Check sheet for the modelled part. Datum: model origin and axes. Units: mm. Round coordinates to 2 decimals unless told otherwise and drop trailing zeros. Order: outer loops, then holes, each group sorted by start corner. A loop starts at its lowest first (then second) coordinate and runs counter-clockwise, first axis right, second up.
Q1. Mould release check, pull along X, two halves, no side actions. Record for faces 1 (the flat face through (1, -2.4, 1)), 2 (the conical face through (1.44, -0.09, -2.52)), 3 (the cylindrical face through (1.2, -1.18, -0.27)): +X half, -X half, draft (parallel to the pull), parting line (faces both ways), or undercut.
Q2. Scan lines: probe 1 along Z at (x, y) = (-1, -1.2); probe 2 along X at (y, z) = (-1, 0.45); probe 3 along Z at (x, y) = (-2.5, -0.9). Record each from-to range of solid material in increasing order.
Q3. Cross-section at A-A on y = -1.1. Record the cut outline in (x, z).
from build123d import *

# Parameters (mm, degrees)
SCHNITT_LINEAR_START            = -1e-07
SCHNITT_LINEAR_AUSTRAGEN1_DEPTH = 2.399991326


# Read off the part's stored shape, not the designer's step: Schnitt-Linear austragen1
with BuildPart() as part:
    # Skizze1 → Basis-Rotation (revolve)
    with BuildSketch(Plane.XY, mode=Mode.PRIVATE) as basis_rotation_sk:
        Polygon((1.2295, 0), (2.75, 0), (3.175426481, -0.245620093), (3.175426481, -2.154379907), (2.75, -2.4), (1.2295, -2.4), align=None)
    revolve(basis_rotation_sk.sketch.rotate(Axis((0, 0, 0), (0, -1, 0)), 90), axis=Axis((0, 0, 0), (0, -1, 0)))

    # Schnitt-Linear austragen1 outline → Schnitt-Linear austragen1 (cut)
    with BuildSketch(Plane.XZ.offset(SCHNITT_LINEAR_START)):
        with BuildLine():
            ThreePointArc((-1.58771324, -2.750000001), (0, -3.175426481), (1.58771324, -2.750000001))
            Line((1.58771324, -2.750000001), (-1.58771324, -2.750000001))
        make_face()
        with BuildLine():
            Line((3.175426481, 0), (1.58771324, -2.750000001))
            ThreePointArc((1.58771324, -2.750000001), (2.75, -1.587713241), (3.175426481, 0))
        make_face()
        with BuildLine():
            ThreePointArc((-3.175426481, 0), (-2.75, -1.587713241), (-1.58771324, -2.750000001))
            Line((-1.58771324, -2.750000001), (-3.175426481, 0))
        make_face()
        with BuildLine():
            Line((1.58771324, 2.750000001), (3.175426481, 0))
            ThreePointArc((3.175426481, 0), (2.75, 1.587713241), (1.58771324, 2.750000001))
        make_face()
        with BuildLine():
            ThreePointArc((-1.58771324, 2.750000001), (-2.75, 1.587713241), (-3.175426481, 0))
            Line((-3.175426481, 0), (-1.58771324, 2.750000001))
        make_face()
        with BuildLine():
            Line((-1.58771324, 2.750000001), (1.58771324, 2.750000001))
            ThreePointArc((1.58771324, 2.750000001), (0, 3.175426481), (-1.58771324, 2.750000001))
        make_face()
    extrude(amount=SCHNITT_LINEAR_AUSTRAGEN1_DEPTH, mode=Mode.SUBTRACT)


solid = part.part
Results found:
1. face 1: draft
1. face 2: +X half
1. face 3: undercut
2. probe 1: z = -2.75 to -0.72, 0.72 to 2.75
2. probe 2: x = -2.92 to -1.14, 1.14 to 2.92
2. probe 3: z = -1.17 to 1.17
3. outline: (-3.18, 0) - (-1.59, -2.75) - (1.59, -2.75) - (3.18, 0) - (1.59, 2.75) - (-1.59, 2.75) - close; hole circle Ø2.46 at (0, 0)
